Verification items for the finished model (mm, model axes). Round coordinates to 2 decimals unless told otherwise and drop trailing zeros. Write each loop counter-clockwise with the first axis right and the second up, starting at its lowest first coordinate (ties: lowest second). Pieces come first, ordered by that corner, then holes. Notation, with made-up numbers: M 69,-15.75 L 117,-15.75 A21 cw 117,18.25 Z; hole C 23,-11 d3. An arc over 180 degrees is marked long. Use a Markdown table: item, result. Add a question column.
from build123d import *

# Parameters (mm, degrees)
SKETCH2_R           = 4
SKETCH2_R_2         = 1.22
BOSS_EXTRUDE2_DEPTH = 3


with BuildPart() as part:
    # Sketch2 → Boss-Extrude2 (new body)
    with BuildSketch(Plane.XY):
        with BuildLine():
            ThreePointArc((-37.264221934, 51.570757137), (-55.048861675, 48.724809542), (-51.528144835, 31.061361936))
            ThreePointArc((-51.528144835, 31.061361936), (-35.404106773, 1.587677725), (-51.528144835, -27.886006485))
            ThreePointArc((-51.528144835, -27.886006485), (-55.048861675, -45.549454092), (-37.264221934, -48.395401687))
            ThreePointArc((-37.264221934, -48.395401687), (-4.021715205, -43.53552404), (17.99893596, -68.90821776))
            ThreePointArc((17.99893596, -68.90821776), (30.213270142, -78.751144089), (42.427604324, -68.90821776))
            ThreePointArc((42.427604324, -68.90821776), (64.448255489, -43.53552404), (97.690762219, -48.395401687))
            ThreePointArc((97.690762219, -48.395401687), (115.475401959, -45.549454092), (111.95468512, -27.886006485))
            ThreePointArc((111.95468512, -27.886006485), (95.830647057, 1.587677725), (111.95468512, 31.061361936))
            ThreePointArc((111.95468512, 31.061361936), (115.475401959, 48.724809542), (97.690762219, 51.570757137))
            ThreePointArc((97.690762219, 51.570757137), (64.448255489, 46.71087949), (42.427604324, 72.08357321))
            ThreePointArc((42.427604324, 72.08357321), (30.213270142, 81.926499539), (17.99893596, 72.08357321))
            ThreePointArc((17.99893596, 72.08357321), (-4.021715205, 46.71087949), (-37.264221934, 51.570757137))
        make_face()
        with Locations((-44.786729858, 41.587677725)):
            Circle(SKETCH2_R, mode=Mode.SUBTRACT)
        with Locations((30.213270142, 69.426499539)):
            Circle(SKETCH2_R, mode=Mode.SUBTRACT)
        with Locations((105.213270142, 41.587677725)):
            Circle(SKETCH2_R, mode=Mode.SUBTRACT)
        with Locations((105.213270142, -38.412322275)):
            Circle(SKETCH2_R, mode=Mode.SUBTRACT)
        with Locations((30.213270142, -66.251144089)):
            Circle(SKETCH2_R, mode=Mode.SUBTRACT)
        with Locations((-44.786729858, -38.412322275)):
            Circle(SKETCH2_R, mode=Mode.SUBTRACT)
        with Locations((30.213270142, 77.926499539)):
            Circle(SKETCH2_R_2, mode=Mode.SUBTRACT)
        with Locations((21.713270142, 69.426499539)):
            Circle(SKETCH2_R_2, mode=Mode.SUBTRACT)
        with Locations((30.213270142, 60.926499539)):
            Circle(SKETCH2_R_2, mode=Mode.SUBTRACT)
        with Locations((38.713270142, 69.426499539)):
            Circle(SKETCH2_R_2, mode=Mode.SUBTRACT)
        with Locations((-40.786729858, 49.087677725)):
            Circle(SKETCH2_R_2, mode=Mode.SUBTRACT)
        with Locations((-37.286729858, 37.587677725)):
            Circle(SKETCH2_R_2, mode=Mode.SUBTRACT)
        with Locations((-48.786729858, 34.087677725)):
            Circle(SKETCH2_R_2, mode=Mode.SUBTRACT)
        with Locations((-52.286729858, 45.587677725)):
            Circle(SKETCH2_R_2, mode=Mode.SUBTRACT)
        with Locations((-37.286729858, -34.412322275)):
            Circle(SKETCH2_R_2, mode=Mode.SUBTRACT)
        with Locations((-48.786729858, -30.912322275)):
            Circle(SKETCH2_R_2, mode=Mode.SUBTRACT)
        with Locations((-40.786729858, -45.912322275)):
            Circle(SKETCH2_R_2, mode=Mode.SUBTRACT)
        with Locations((-52.286729858, -42.412322275)):
            Circle(SKETCH2_R_2, mode=Mode.SUBTRACT)
        with Locations((112.713270142, -42.412322275)):
            Circle(SKETCH2_R_2, mode=Mode.SUBTRACT)
        with Locations((101.213270142, -45.912322275)):
            Circle(SKETCH2_R_2, mode=Mode.SUBTRACT)
        with Locations((97.713270142, -34.412322275)):
            Circle(SKETCH2_R_2, mode=Mode.SUBTRACT)
        with Locations((109.213270142, -30.912322275)):
            Circle(SKETCH2_R_2, mode=Mode.SUBTRACT)
        with Locations((97.713270142, 37.587677725)):
            Circle(SKETCH2_R_2, mode=Mode.SUBTRACT)
        with Locations((109.213270142, 34.087677725)):
            Circle(SKETCH2_R_2, mode=Mode.SUBTRACT)
        with Locations((101.213270142, 49.087677725)):
            Circle(SKETCH2_R_2, mode=Mode.SUBTRACT)
        with Locations((112.713270142, 45.587677725)):
            Circle(SKETCH2_R_2, mode=Mode.SUBTRACT)
        with Locations((30.213270142, -57.751144089)):
            Circle(SKETCH2_R_2, mode=Mode.SUBTRACT)
        with Locations((38.713270142, -66.251144089)):
            Circle(SKETCH2_R_2, mode=Mode.SUBTRACT)
        with Locations((21.713270142, -66.251144089)):
            Circle(SKETCH2_R_2, mode=Mode.SUBTRACT)
        with Locations((30.213270142, -74.751144089)):
            Circle(SKETCH2_R_2, mode=Mode.SUBTRACT)
    extrude(amount=BOSS_EXTRUDE2_DEPTH)


solid = part.part
1. Cross-section at A-A on y = 16. Enter the section's corners in (x, z), plus the area to 3 significant figures.
2. Cross-section at C-C on z = 1.85. Count the separate pieces of the cut face and the enclosed holes in it, plus the area to 3 significant figures.
3. Release check for a two-part mould opening along X. For faces 1 (the cylindrical face through (-40.97, -37.21, 1.48)), 2 (the cylindrical face through (-54.89, 48.95, 1.48)), 3 (the cylindrical face through (-35.408, 2.078, 1.479)), 4 (the flat face through (29, 3, 3)) record: +X half, -X half, draft (parallel to the pull), parting line (faces both ways), or undercut.
4. Depth check by flat-ended pin: pin 1 Ø4 at (x, y) = (38.71, 69.43) entering from +Z; pin 2 Ø1 at (x, z) = (-9, 1) entering from +Y. Enter the tip coordinate at first touch or a pass-through.
5. Scan lines: line 1 along X through (y, z) = (50.5, 1.9); line 2 along X through (y, z) = (47.5, 1.25); line 3 along X through (y, z) = (-5, 0.7). Record each from-to range of solid material in increasing order. Write a range as from..to.
6. Cross-section at B-B on x = 92. Enter the section's corners in (y, z), plus the area to 3 significant figures.
Answer:
| question | item | result |
|---|---|---|
| 1 | outline | M -38.51,0 L 98.94,0 L 98.94,3 L -38.51,3 Z |
| 1 | area | 412 mm^2 |
| 2 | separate pieces | 1 |
| 2 | enclosed holes | 30 |
| 2 | area | 16,000 mm^2 |
| 3 | face 1 | undercut |
| 3 | face 2 | undercut |
| 3 | face 3 | -X half |
| 3 | face 4 | draft |
| 4 | pin 1 | stops at z = 3 |
| 4 | pin 2 | stops at y = 45.38 |
| 5 | line 1 | x = -53.55..-35.76, 3.36..57.07, 96.19..113.98 |
| 5 | line 2 | x = -55.8..-30.33, -2.08..62.5, 90.75..116.23 |
| 5 | line 3 | x = -36.03..96.46 |
| 6 | outline | M -44.9,0 L 48.08,0 L 48.08,3 L -44.9,3 Z |
| 6 | area | 279 mm^2 |
